The listing builds one solid part. Answer for the finished solid, in the listing's coordinates (mm). A direction names the side the tool comes from. Give positions to 0.01 mm unless a question says otherwise; leave off trailing zeros. Write each loop counter-clockwise with the first axis right and the second up, starting at its lowest first coordinate (ties: lowest second). Pieces come first, ordered by that corner, then holes. Notation, with made-up numbers: (-32, 78) - (-3, 78) arc R25 ccw to (-3, 107) - close; hole circle Ø5 at (-36, 15.25). An arc over 180 degrees is marked (long way). Write each question's results on one line, items separated by ' | '. Start each with the question number.
Q1. Flat-ended cylindrical pins translate along their axes: pin 1 Ø3 at (x, y) = (-63.5, 25.4) entering from -Z; pin 2 Ø1.6 at (x, y) = (63.5, -25.4) entering from -Z (3 decimals); pin 3 Ø10 at (y, z) = (16.5, 27.5) entering from -X; pin 4 Ø6 at (x, y) = (22, 19.5) entering from +Z (3 decimals). Find the tip coordinate at first contact, or state that the pin passes through.
Q2. For faces 5 (the face through (-3.9, 12.3, 48.889)), 6 (the face through (-4.08, -18.373, 53.037)), 7 (the face through (0, 0, 60.325)), determine the directions among +Z, -Z, +X, -X, +Y, -Y from which every point of the face is accessible in a straight line to the end or side of a thin tool.
Q3. Find the intervals of material crossed by probe 1 along X at (y, z) = (25.4, 5); probe 2 along Y at (x, z) = (63.5, 3.75); probe 3 along X at (y, z) = (-25, 1), in increasing order.
Q4. Section D-D (y = -15.5) is taken. State how many separate pieces and enclosed holes the cut face has, plus the area to 3 significant figures.
Q5. For a pull along Y with two mould halves and no side action, classify faces 1 (the face through (-4.08, -18.373, 39.829)), 2 (the face through (64.67, -26.3, 6.74)), 3 (the face through (-3.9, 12.3, 45.587)), 4 (the face through (62.706, 26.645, 6.738)) as pulls with the +Y half, pulls with the -Y half, needs draft (parallel to the pull), parting line crosses it, or undercut.
Q6. Section A-A (z = 13) is taken. Determine the outline of the cut face in (x, y).
Q7. Section C-C (x = -42) is taken. Determine the outline of the cut face in (y, z) (3 decimals), plus the area to 3 significant figures.
Q8. Section B-B (y = 32) is taken. Determine the outline of the cut face in (x, z) (3 decimals).
```python
from build123d import *

# Parameters (mm, degrees)
F0_W           = 152.4
F0_H           = 76.2
F1_DEPTH       = 9.525
F3_D           = 2.7051
F3_CSINK_D     = 7.7978
F3_CSINK_ANGLE = 82
F4_R           = 18.8204674016
F5_DEPTH       = 50.8
F6_W           = 14.3435228881
F6_H           = 1.5875


# Not quite as in the source:
# - a fillet or chamfer that OpenCascade refuses, or shapes differently, is made with other operations: its cross-section is extruded or revolved along the edge and cut away or added


with BuildPart() as f1:
    # F0 (on Top) → F1 (new body)
    with BuildSketch(Plane.XY):
        Rectangle(F0_W, F0_H)
    extrude(amount=F1_DEPTH)

    # F3 (through all)
    with Locations(Plane.XY.offset(9.525)):
        with Locations((-63.5, 25.4), (63.5, 25.4), (-63.5, -25.4), (63.5, -25.4)):
            CounterSinkHole(F3_D / 2, F3_CSINK_D / 2, counter_sink_angle=F3_CSINK_ANGLE)

    # F4 (on face) → F5 (join)
    with BuildSketch(Plane.XY.offset(9.525)):
        Circle(F4_R)
    extrude(amount=F5_DEPTH)

    # F6 (on Front) → F7 (revolve, cut)
    with BuildSketch(Plane.XZ):
        with Locations((19.8717614441, 34.8877100782)):
            Rectangle(F6_W, F6_H)
        with Locations((19.8717614441, 38.1897100782)):
            Rectangle(F6_W, F6_H)
        with Locations((19.8717614441, 41.4917100782)):
            Rectangle(F6_W, F6_H)
        with Locations((19.8717614441, 44.7937100782)):
            Rectangle(F6_W, F6_H)
        with Locations((19.8717614441, 48.0957100782)):
            Rectangle(F6_W, F6_H)
        with Locations((19.8717614441, 51.3977100782)):
            Rectangle(F6_W, F6_H)
        with Locations((19.8717614441, 54.6997100782)):
            Rectangle(F6_W, F6_H)
        with Locations((19.8717614441, 58.0017100782)):
            Rectangle(F6_W, F6_H)
    revolve(axis=Axis((0, 0, 9.525), (0, 0, -1)), mode=Mode.SUBTRACT)

    # F8: chamfer of 1.5875 on 2 edges, made by hand

    # F8_s1 → F8_t2 (revolve)
    with BuildSketch(Plane.XZ):
        Polygon((20.4079674016, 9.525), (18.8204674016, 11.1125), (18.8204674016, 9.525), align=None)
    revolve(axis=Axis((0, 0, 9.525), (0, 0, 1)))

    # F8_s3 → F8_t4 (revolve, cut)
    with BuildSketch(Plane.XZ):
        Polygon((18.8204674016, 58.7375), (17.2329674016, 60.325), (18.8204674016, 60.325), align=None)
    revolve(axis=Axis((0, 0, 60.325), (0, 0, 1)), mode=Mode.SUBTRACT)


solid = f1.part
```
Answers below:
1) pin 1: stops at z = 0 | pin 2: passes through | pin 3: stops at x = -14.9 | pin 4: stops at z = 9.525
2) face 5: none | face 6: +Z | face 7: +Z, +X, -X, +Y, -Y
3) probe 1: x = -76.2 to -64.85, -62.15 to 62.15, 64.85 to 76.2 | probe 2: y = -38.1 to -26.75, -24.05 to 24.05, 26.75 to 38.1 | probe 3: x = -76.2 to -64.79, -62.21 to 62.21, 64.79 to 76.2
4) separate pieces: 9 | enclosed holes: 0 | area: 2,260 mm2
5) face 1: parting line crosses it | face 2: undercut | face 3: needs draft | face 4: undercut
6) outline: circle Ø37.64 at (0, 0)
7) outline: (-38.1, 0) - (38.1, 0) - (38.1, 9.525) - (-38.1, 9.525) - close | area: 726 mm2
8) outline: (-76.2, 0) - (76.2, 0) - (76.2, 9.525) - (-76.2, 9.525) - close
